Geometry: final body of the model. Coordinates: model frame, mm. A direction names the side the tool comes from. Give positions to 0.01 mm unless a question says otherwise; leave off trailing zeros. Order: outer loops, then holes, each group sorted by start corner. A loop starts at its lowest first (then second) coordinate and runs counter-clockwise, first axis right, second up. Notation, with made-up numbers: (63.5, 78.5) -> (79.5, 78.5) arc R22 ccw to (79.5, 86.5) -> close; hole circle Ø1 at (54.25, 65). An arc over 180 degrees is marked (long way). One line per question, with ' | ' between items. Start each with the question number.
(1) First-contact query: pin 1 Ø1.5 at (x, y) = (22, -266) entering from +Z; pin 2 Ø6 at (y, z) = (-262.5, -299) entering from -X; pin 3 Ø1.3 at (x, z) = (16.04, -270.55) entering from -Y. Flat tips, straight axial feed; report the tip coordinate or a pass-through.
(2) Section A-A (x = -35). Return loops of the section in (y, z) (3 decimals).
(3) Section B-B (z = -297). Return loops of the section in (x, y).
(4) Mould query, pull axis X, two halves, no side actions, for faces 1 (the face through (3.4, -288.5, -309.75)), 2 (the face through (20.16, -264.96, -268.7)), 3 (the face through (19, -296, -273)), 4 (the face through (-1, -284, -313.5)). Classes: +X half, -X half, draft (parallel to the pull), parting line (faces both ways), or undercut.
(5) Section C-C (y = -296.5). Return loops of the section in (x, z) (3 decimals).
(6) Ray query, L1, parallel to Y at x = 15, z = -259 (3 decimals); L2, parallel to X at y = -315, z = -311.2 (3 decimals); L3, parallel to X at y = -288.5, z = -311.65. Return the intervals inside material, ascending.
(7) Set-up query: faces 5 (the face through (16.5, -265, -282)), 6 (the face through (17, -267.5, -296)), 7 (the face through (5, -288.6, -309.4)), 8 (the face through (20, -265, -263)), 9 (the face through (11, -296, -273)). Return all of +Z, -Z, +X, -X, +Y, -Y with unobstructed straight access to the full face (end or side cutting, diameter ignored); none if empty.
(8) Section D-D (z = -278). Return loops of the section in (x, y), then the cut area to 3 significant figures.
```python
from build123d import *

# Parameters (mm, degrees)
EXTRUDE031_DEPTH = 5
SKETCH021_R      = 1.125
EXTRUDE005_DEPTH = 5
SKETCH020_W      = 8
SKETCH020_H      = 25.5
SKETCH020_R      = 1.625
EXTRUDE004_DEPTH = 5
SKETCH019_R      = 1.125
EXTRUDE003_DEPTH = 5
SKETCH093_W      = 82
SKETCH093_H      = 72
SKETCH093_R      = 1.625
EXTRUDE030_DEPTH = 4.5


with BuildPart() as obj1:
    # Sketch094 → Extrude031 (new body)
    with BuildSketch(Plane.XY):
        with BuildLine():
            ThreePointArc((-7.5, -283.5), (-12.5, -288.5), (-7.5, -293.5))
            Line((-7.5, -293.5), (0, -293.5))
            ThreePointArc((0, -293.5), (5, -288.5), (0, -283.5))
            Line((0, -283.5), (-7.5, -283.5))
        make_face()
    extrude(amount=EXTRUDE031_DEPTH)


with BuildPart() as obj1_1:
    # Extrude031 placement: moved
    add(obj1.part.moved(Location((0, 0, -309.75))))


with BuildPart() as obj2:
    # Sketch021 (on Extrude) → Extrude005 (new body)
    with BuildSketch(Plane.XZ):
        Polygon((-25, -309), (-25, -301), (16.5, -301), (16.5, -263), (24.5, -263), (24.5, -309), align=None)
        with Locations((-20.4, -304.4)):
            Circle(SKETCH021_R, mode=Mode.SUBTRACT)
        with Locations((20.4, -267.6)):
            Circle(SKETCH021_R, mode=Mode.SUBTRACT)
    extrude(amount=EXTRUDE005_DEPTH)


with BuildPart() as obj2_1:
    # Extrude005 placement: moved
    add(obj2.part.moved(Location((0, -262.5, 0))))


with BuildPart() as gpshold:
    # Sketch020 → Extrude004 (new body)
    with BuildSketch(Plane.XY.offset(-263)):
        with Locations((15, -294.25)):
            Rectangle(SKETCH020_W, SKETCH020_H)
        with Locations((15, -284.1)):
            Circle(SKETCH020_R, mode=Mode.SUBTRACT)
        with Locations((15, -304.5)):
            Circle(SKETCH020_R, mode=Mode.SUBTRACT)
    extrude(amount=EXTRUDE004_DEPTH)


with BuildPart() as obj3:
    # Sketch019 → Extrude003 (new body)
    with BuildSketch(Plane.XZ.offset(295)):
        Polygon((28, -309), (28, -301), (19, -301), (19, -263), (11, -263), (11, -301), (-13, -301), (-13, -284), (-19, -284), (-19, -309), align=None)
        with Locations((-15.96, -286.8)):
            Circle(SKETCH019_R, mode=Mode.SUBTRACT)
        with Locations((-0.15, -304.37)):
            Circle(SKETCH019_R, mode=Mode.SUBTRACT)
        with Locations((20.15, -304.37)):
            Circle(SKETCH019_R, mode=Mode.SUBTRACT)
        with Locations((16.04, -270.55)):
            Circle(SKETCH019_R, mode=Mode.SUBTRACT)
    extrude(amount=EXTRUDE003_DEPTH)


with BuildPart() as base012:
    # Sketch093 → Extrude030 (new body)
    with BuildSketch(Plane.XY):
        with Locations((0, -285)):
            Rectangle(SKETCH093_W, SKETCH093_H)
        with Locations((-35, -315)):
            Circle(SKETCH093_R, mode=Mode.SUBTRACT)
        with Locations((35, -315)):
            Circle(SKETCH093_R, mode=Mode.SUBTRACT)
        with Locations((35, -255)):
            Circle(SKETCH093_R, mode=Mode.SUBTRACT)
        with Locations((-35, -255)):
            Circle(SKETCH093_R, mode=Mode.SUBTRACT)
        with BuildLine():
            ThreePointArc((-3.658125, -285.3), (-12.5, -288.5), (-3.658125, -291.7))
            Line((-3.658125, -291.7), (-0.399218, -291.675))
            ThreePointArc((-0.399218, -291.675), (3.2, -288.5), (-0.399218, -285.325))
            Line((-0.399218, -285.325), (-3.658125, -285.3))
        make_face(mode=Mode.SUBTRACT)
    extrude(amount=EXTRUDE030_DEPTH)


with BuildPart() as base012_1:
    # Extrude030 placement: moved
    add(base012.part.moved(Location((0, 0, -313.5))))

    # Fusion078: union obj2, gpsHold, obj3
    add(obj2_1.part)
    add(gpshold.part)
    add(obj3.part)

    # Cut035: cut obj1
    add(obj1_1.part, mode=Mode.SUBTRACT)


solid = base012_1.part
```
Response:
1) pin 1: stops at z = -263 | pin 2: stops at x = -25 | pin 3: stops at y = -267.5
2) outline: (-321, -313.5) -> (-316.625, -313.5) -> (-316.625, -309) -> (-321, -309) -> close; (-313.375, -313.5) -> (-256.625, -313.5) -> (-256.625, -309) -> (-313.375, -309) -> close; (-253.375, -313.5) -> (-249, -313.5) -> (-249, -309) -> (-253.375, -309) -> close
3) outline: (-19, -300) -> (-13, -300) -> (-13, -295) -> (-19, -295) -> close; (11, -300) -> (19, -300) -> (19, -295) -> (11, -295) -> close; (16.5, -267.5) -> (24.5, -267.5) -> (24.5, -262.5) -> (16.5, -262.5) -> close
4) face 1: undercut | face 2: undercut | face 3: +X half | face 4: draft
5) outline: (-41, -313.5) -> (41, -313.5) -> (41, -309) -> (28, -309) -> (28, -301) -> (19, -301) -> (19, -258) -> (11, -258) -> (11, -301) -> (-13, -301) -> (-13, -284) -> (-19, -284) -> (-19, -309) -> (-41, -309) -> close; hole circle Ø2.25 at (-15.96, -286.8); hole circle Ø2.25 at (-0.15, -304.37); hole circle Ø2.25 at (16.04, -270.55); hole circle Ø2.25 at (20.15, -304.37)
6) L1: y = -307 to -306.125, -302.875 to -285.725, -282.475 to -281.5 | L2: x = -41 to -36.625, -33.375 to 33.375, 36.625 to 41 | L3: x = -41 to -12.5, 3.2 to 41
7) face 5: +Z, -X, +Y | face 6: +Z, +X, -X | face 7: +Z | face 8: +Z, +X, -X, +Y | face 9: +Z, +Y, -Y
8) outline: (11, -300) -> (19, -300) -> (19, -295) -> (11, -295) -> close; (16.5, -267.5) -> (24.5, -267.5) -> (24.5, -262.5) -> (16.5, -262.5) -> close | area: 80.0 mm^2
